Work out the finished part from the listing and answer in its coordinate system (mm). A direction names the side the tool comes from. Coordinates: 2 decimals unless noted, no trailing zeros. Use a Markdown table: item, result.
from build123d import *

# Parameters (mm, degrees)
SKETCH1_R           = 4.826
SKETCH1_R_2         = 14.28115
SKETCH1_R_3         = 3.3528
SKETCH1_R_4         = 4.953
SKETCH1_R_5         = 3.3782
SKETCH1_R_6         = 2.5527
SKETCH1_R_7         = 5.5626
BOSS_EXTRUDE1_DEPTH = 4.7625


with BuildPart() as part:
    # Sketch1 → Boss-Extrude1 (new body)
    with BuildSketch(Plane.XZ):
        with BuildLine():
            Line((3.338142419, -25.866609912), (66.074894217, -94.306702782))
            ThreePointArc((66.074894217, -94.306702782), (70.322928635, -97.34992205), (75.436751798, -98.425))
            Line((75.436751798, -98.425), (514.35, -98.425))
            ThreePointArc((514.35, -98.425), (523.330256121, -94.705256121), (527.05, -85.725))
            Line((527.05, -85.725), (527.05, -12.7))
            ThreePointArc((527.05, -12.7), (523.330256121, -3.719743879), (514.35, 0))
            Line((514.35, 0), (12.7, 0))
            ThreePointArc((12.7, 0), (3.719743879, -3.719743879), (0, -12.7))
            Line((0, -12.7), (0, -17.28490713))
            ThreePointArc((0, -17.28490713), (0.863919752, -21.888949307), (3.338142419, -25.866609912))
        make_face()
        with Locations((34.925, -19.05)):
            Circle(SKETCH1_R, mode=Mode.SUBTRACT)
        with Locations((476.25, -19.05)):
            Circle(SKETCH1_R, mode=Mode.SUBTRACT)
        with Locations((19.05, -19.05)):
            Circle(SKETCH1_R, mode=Mode.SUBTRACT)
        with Locations((247.65, -15.24)):
            Circle(SKETCH1_R, mode=Mode.SUBTRACT)
        with Locations((369.99417663, -38.1)):
            Circle(SKETCH1_R_2, mode=Mode.SUBTRACT)
        with Locations((314.41897663, -7.9248)):
            Circle(SKETCH1_R_3, mode=Mode.SUBTRACT)
        with Locations((425.56937663, -7.9248)):
            Circle(SKETCH1_R_3, mode=Mode.SUBTRACT)
        with Locations((73.025, -82.55)):
            Circle(SKETCH1_R_4, mode=Mode.SUBTRACT)
        with Locations((95.25, -12.7)):
            Circle(SKETCH1_R_5, mode=Mode.SUBTRACT)
        with Locations((95.25, -85.725)):
            Circle(SKETCH1_R_5, mode=Mode.SUBTRACT)
        with Locations((146.05, -12.7)):
            Circle(SKETCH1_R_5, mode=Mode.SUBTRACT)
        with Locations((146.05, -85.725)):
            Circle(SKETCH1_R_5, mode=Mode.SUBTRACT)
        with Locations((171.45, -12.7)):
            Circle(SKETCH1_R_5, mode=Mode.SUBTRACT)
        with Locations((171.45, -85.725)):
            Circle(SKETCH1_R_5, mode=Mode.SUBTRACT)
        with Locations((196.85, -12.7)):
            Circle(SKETCH1_R_5, mode=Mode.SUBTRACT)
        with Locations((196.85, -85.725)):
            Circle(SKETCH1_R_5, mode=Mode.SUBTRACT)
        with Locations((222.25, -12.7)):
            Circle(SKETCH1_R_5, mode=Mode.SUBTRACT)
        with Locations((222.25, -85.725)):
            Circle(SKETCH1_R_5, mode=Mode.SUBTRACT)
        with Locations((247.65, -85.725)):
            Circle(SKETCH1_R_5, mode=Mode.SUBTRACT)
        with Locations((273.05, -12.7)):
            Circle(SKETCH1_R_5, mode=Mode.SUBTRACT)
        with Locations((273.05, -85.725)):
            Circle(SKETCH1_R_5, mode=Mode.SUBTRACT)
        with Locations((298.45, -12.7)):
            Circle(SKETCH1_R_5, mode=Mode.SUBTRACT)
        with Locations((298.45, -85.725)):
            Circle(SKETCH1_R_5, mode=Mode.SUBTRACT)
        with Locations((323.85, -85.725)):
            Circle(SKETCH1_R_5, mode=Mode.SUBTRACT)
        with Locations((349.25, -12.7)):
            Circle(SKETCH1_R_5, mode=Mode.SUBTRACT)
        with Locations((349.25, -85.725)):
            Circle(SKETCH1_R_5, mode=Mode.SUBTRACT)
        with Locations((374.65, -12.7)):
            Circle(SKETCH1_R_5, mode=Mode.SUBTRACT)
        with Locations((374.65, -85.725)):
            Circle(SKETCH1_R_5, mode=Mode.SUBTRACT)
        with Locations((400.05, -12.7)):
            Circle(SKETCH1_R_5, mode=Mode.SUBTRACT)
        with Locations((400.05, -85.725)):
            Circle(SKETCH1_R_5, mode=Mode.SUBTRACT)
        with Locations((425.45, -85.725)):
            Circle(SKETCH1_R_5, mode=Mode.SUBTRACT)
        with Locations((450.85, -12.7)):
            Circle(SKETCH1_R_5, mode=Mode.SUBTRACT)
        with Locations((450.85, -85.725)):
            Circle(SKETCH1_R_5, mode=Mode.SUBTRACT)
        with Locations((476.25, -85.725)):
            Circle(SKETCH1_R_5, mode=Mode.SUBTRACT)
        with Locations((501.65, -12.7)):
            Circle(SKETCH1_R_5, mode=Mode.SUBTRACT)
        with Locations((501.65, -85.725)):
            Circle(SKETCH1_R_5, mode=Mode.SUBTRACT)
        with Locations((123.825, -19.05)):
            Circle(SKETCH1_R_6, mode=Mode.SUBTRACT)
        with Locations((114.3, -28.575)):
            Circle(SKETCH1_R_6, mode=Mode.SUBTRACT)
        with Locations((133.35, -9.525)):
            Circle(SKETCH1_R_6, mode=Mode.SUBTRACT)
        with Locations((114.3, -88.9)):
            Circle(SKETCH1_R_6, mode=Mode.SUBTRACT)
        with Locations((123.825, -79.375)):
            Circle(SKETCH1_R_6, mode=Mode.SUBTRACT)
        with Locations((133.35, -69.85)):
            Circle(SKETCH1_R_6, mode=Mode.SUBTRACT)
        with Locations((331.25917663, -40.8178)):
            Circle(SKETCH1_R_7, mode=Mode.SUBTRACT)
        with Locations((408.72917663, -66.2178)):
            Circle(SKETCH1_R_7, mode=Mode.SUBTRACT)
        with Locations((331.25917663, -66.2178)):
            Circle(SKETCH1_R_7, mode=Mode.SUBTRACT)
        with Locations((408.72917663, -40.8178)):
            Circle(SKETCH1_R_7, mode=Mode.SUBTRACT)
        with Locations((69.85, -12.7)):
            Circle(SKETCH1_R_5, mode=Mode.SUBTRACT)
        with Locations((51.950539741, -57.756517342)):
            Circle(SKETCH1_R_5, mode=Mode.SUBTRACT)
        with BuildLine():
            Line((49.23354708, -22.225), (85.725, -22.225))
            ThreePointArc((85.725, -22.225), (90.215128061, -24.084871939), (92.075, -28.575))
            Line((92.075, -28.575), (92.075, -69.241869017))
            ThreePointArc((92.075, -69.241869017), (90.041376556, -72.204618509), (86.545623901, -71.37201882))
            Line((86.545623901, -71.37201882), (46.879170981, -27.530149804))
            ThreePointArc((46.879170981, -27.530149804), (46.33149172, -24.112094846), (49.23354708, -22.225))
        make_face(mode=Mode.SUBTRACT)
        with BuildLine():
            Line((174.53102337, -76.2), (153.9875, -76.2))
            ThreePointArc((153.9875, -76.2), (151.74243597, -75.27006403), (150.8125, -73.025))
            Line((150.8125, -73.025), (150.8125, -25.4))
            ThreePointArc((150.8125, -25.4), (151.74243597, -23.15493597), (153.9875, -22.225))
            Line((153.9875, -22.225), (174.53102337, -22.225))
            ThreePointArc((174.53102337, -22.225), (176.7760874, -23.15493597), (177.70602337, -25.4))
            Line((177.70602337, -25.4), (177.70602337, -73.025))
            ThreePointArc((177.70602337, -73.025), (176.7760874, -75.27006403), (174.53102337, -76.2))
        make_face(mode=Mode.SUBTRACT)
        with BuildLine():
            Line((227.625953961, -27.542449226), (192.749212716, -65.68702112))
            ThreePointArc((192.749212716, -65.68702112), (189.25689352, -66.504322828), (187.23102337, -63.544571894))
            Line((187.23102337, -63.544571894), (187.23102337, -25.4))
            ThreePointArc((187.23102337, -25.4), (188.16095934, -23.15493597), (190.40602337, -22.225))
            Line((190.40602337, -22.225), (225.282764614, -22.225))
            ThreePointArc((225.282764614, -22.225), (228.188182079, -24.119697554), (227.625953961, -27.542449226))
        make_face(mode=Mode.SUBTRACT)
        with BuildLine():
            Line((252.4125, -73.025), (252.4125, -33.144184818))
            ThreePointArc((252.4125, -33.144184818), (254.43837015, -30.184433885), (257.930689347, -31.001735592))
            Line((257.930689347, -31.001735592), (294.394930591, -70.882550774))
            ThreePointArc((294.394930591, -70.882550774), (294.957158709, -74.305302446), (292.051741244, -76.2))
            Line((292.051741244, -76.2), (255.5875, -76.2))
            ThreePointArc((255.5875, -76.2), (253.34243597, -75.27006403), (252.4125, -73.025))
        make_face(mode=Mode.SUBTRACT)
        with BuildLine():
            Line((239.7125, -76.2), (203.248258756, -76.2))
            ThreePointArc((203.248258756, -76.2), (200.342841291, -74.305302446), (200.905069409, -70.882550774))
            Line((200.905069409, -70.882550774), (237.369310653, -31.001735592))
            ThreePointArc((237.369310653, -31.001735592), (240.86162985, -30.184433885), (242.8875, -33.144184818))
            Line((242.8875, -33.144184818), (242.8875, -73.025))
            ThreePointArc((242.8875, -73.025), (241.95756403, -75.27006403), (239.7125, -76.2))
        make_face(mode=Mode.SUBTRACT)
        with BuildLine():
            Line((270.017235386, -22.225), (304.89397663, -22.225))
            ThreePointArc((304.89397663, -22.225), (307.13904066, -23.15493597), (308.06897663, -25.4))
            Line((308.06897663, -25.4), (308.06897663, -63.544571894))
            ThreePointArc((308.06897663, -63.544571894), (306.04310648, -66.504322828), (302.550787284, -65.68702112))
            Line((302.550787284, -65.68702112), (267.674046039, -27.542449226))
            ThreePointArc((267.674046039, -27.542449226), (267.111817921, -24.119697554), (270.017235386, -22.225))
        make_face(mode=Mode.SUBTRACT)
        with BuildLine():
            Line((433.50687663, -22.225), (461.453022572, -22.225))
            ThreePointArc((461.453022572, -22.225), (464.297387539, -23.989250932), (463.980698305, -27.321322562))
            Line((463.980698305, -27.321322562), (436.034552363, -64.087036098))
            ThreePointArc((436.034552363, -64.087036098), (432.493157106, -65.174533525), (430.33187663, -62.165713536))
            Line((430.33187663, -62.165713536), (430.33187663, -25.4))
            ThreePointArc((430.33187663, -25.4), (431.2618126, -23.15493597), (433.50687663, -22.225))
        make_face(mode=Mode.SUBTRACT)
        with BuildLine():
            Line((442.665404361, -71.103677438), (465.784824267, -40.687963902))
            ThreePointArc((465.784824267, -40.687963902), (469.326219524, -39.600466475), (471.4875, -42.609286464))
            Line((471.4875, -42.609286464), (471.4875, -73.025))
            ThreePointArc((471.4875, -73.025), (470.55756403, -75.27006403), (468.3125, -76.2))
            Line((468.3125, -76.2), (445.193080094, -76.2))
            ThreePointArc((445.193080094, -76.2), (442.348715126, -74.435749068), (442.665404361, -71.103677438))
        make_face(mode=Mode.SUBTRACT)
    extrude(amount=-BOSS_EXTRUDE1_DEPTH)


solid = part.part
(1) Given P1, Ø1.4, axis at y = 1.5, z = -64, coming from the -X side; P2, Ø1.5, axis at y = 3.5, z = -20, coming from the -X side, each flat-ended and moving along its own axis, determine where each tip first touches the part or whether it passes through.
Conclusion:
| item | result |
|---|---|
| P1 | x = 37.65 |
| P2 | x = 0.15 |
(2) A cutting plane is placed at A-A (y = 1.2). Give the number of separate pieces and of enclosed holes in the cut face, then the cut area to 3 significant figures.
Conclusion:
| item | result |
|---|---|
| separate pieces | 1 |
| enclosed holes | 56 |
| area | 37,500 mm2 |
(3) Straight lines are drawn through the part: L1, parallel to Z at x = 330.5, y = 4.5 (3 decimals); L2, parallel to Z at x = 133.35, y = 3 (3 decimals); L3, parallel to Z at x = 172, y = 4.45 (3 decimals). For each, find the intervals that lie inside material, in ascending order.
Conclusion:
| item | result |
|---|---|
| L1 | -98.425 to -71.728, -60.707 to -46.328, -35.307 to 0 |
| L2 | -98.425 to -72.403, -67.297 to -12.078, -6.972 to 0 |
| L3 | -98.425 to -89.058, -82.392 to -76.2, -22.225 to -16.033, -9.367 to 0 |
(4) Determine the mould class of faces 3 (the cylindrical face through (523.43, 2.35, -3.82)), 4 (the flat face through (454.06, 2.35, -56.11)), 5 (the flat face through (34.27, 2.35, -59.61)) for opening direction X: pulls with the +X half, pulls with the -X half, needs draft (parallel to the pull), parting line crosses it, or undercut.
Conclusion:
| item | result |
|---|---|
| face 3 | pulls with the +X half |
| face 4 | undercut |
| face 5 | pulls with the -X half |
(5) Which of the six approach directions +Z, -Z, +X, -X, +Y, -Y give full straight-line access (tool end or side, diameter ignored) to faces 1 (the flat face through (260, 4.762, -27)), 2 (the flat face through (285.357, 2.348, -46.882))?
Conclusion:
| item | result |
|---|---|
| face 1 | +Z, -Z, +X, -X, +Y |
| face 2 | +Y, -Y |
